Source: CAD feature listing. Evaluate the final solid. Frame: model axes, mm. Give positions to 0.01 mm unless a question says otherwise; leave off trailing zeros. Loops run counter-clockwise (first coordinate to the right, second up) from the corner with the lowest first, then second, coordinate; pieces in that order, holes last. Notation, with made-up numbers: (63.5, 32) - (109.5, 32) arc R28 cw to (109.5, 54) - close; hole circle Ø6 at (-2, 27). An arc over 180 degrees is marked (long way). Write each question's results on one line, items separated by ' | '. Start each with the question number.
(1) Cut plane C-C on x = 182.5. Return the cut outline in (y, z), then the cut area to 3 significant figures.
(2) Cut plane A-A on y = -4. Return the cut outline in (x, z), then the cut area to 3 significant figures.
(3) Material intervals for line 1 along Z through (x, y) = (131, 2.75); line 2 along X through (y, z) = (0.25, -221); line 3 along X through (y, z) = (6.75, -209.5), sorted ascending. Write a range as [from, to].
(4) Cut plane B-B on z = -172. Return the cut outline in (x, y), then the cut area to 3 significant figures.
(5) Contact query for flat-ended pins moving along their axis: pin 1 (5 mm diameter, centred on y = 7, z = -216.5, fed in from +X); pin 2 (3 mm diameter, centred on x = 78, y = 2, fed in from -Z); pin 3 (5 mm diameter, centred on y = 6, z = -40, fed in from -X); pin 4 (8 mm diameter, centred on y = 3.5, z = -171.5, fed in from -X). Output: stop coordinate, or through.
from build123d import *

# Parameters (mm, degrees)
SKETCH1_W           = 220
SKETCH1_H           = 300
BOSS_EXTRUDE1_DEPTH = 10
FILLET1_R           = 30
SKETCH9_W           = 15
SKETCH9_H           = 10
CUT_EXTRUDE1_DEPTH  = 10
SKETCH8_W           = 15
SKETCH8_H           = 10
CUT_EXTRUDE2_DEPTH  = 10
BOSS_EXTRUDE3_DEPTH = 10


with BuildPart() as part:
    # Sketch1 → Boss-Extrude1 (new body)
    with BuildSketch(Plane(origin=(0, 0, 0), x_dir=(1, 0, 0), z_dir=(0, 1, 0))):
        with Locations((110, 150)):
            Rectangle(SKETCH1_W, SKETCH1_H)
    extrude(amount=BOSS_EXTRUDE1_DEPTH)

    # Fillet1
    fillet1_edges = [part.edges().sort_by_distance(p)[0] for p in [
        (0, 5, -300),
        (220, 5, -300),
        (220, 5, 0),
        (0, 5, 0),
    ]]
    fillet(fillet1_edges, radius=FILLET1_R)

    # Sketch9 → Cut-Extrude1 (cut)
    with BuildSketch(Plane(origin=(220, 0, 0), x_dir=(0, 0, -1), z_dir=(1, 0, 0))):
        with Locations((262.5, 5)):
            Rectangle(SKETCH9_W, SKETCH9_H)
        with Locations((232.5, 5)):
            Rectangle(SKETCH9_W, SKETCH9_H)
        with Locations((202.5, 5)):
            Rectangle(SKETCH9_W, SKETCH9_H)
        with Locations((172.5, 5)):
            Rectangle(SKETCH9_W, SKETCH9_H)
        with Locations((142.5, 5)):
            Rectangle(SKETCH9_W, SKETCH9_H)
        with Locations((112.5, 5)):
            Rectangle(SKETCH9_W, SKETCH9_H)
        with Locations((82.5, 5)):
            Rectangle(SKETCH9_W, SKETCH9_H)
        with Locations((52.5, 5)):
            Rectangle(SKETCH9_W, SKETCH9_H)
    extrude(amount=-CUT_EXTRUDE1_DEPTH, mode=Mode.SUBTRACT)

    # Sketch8 → Cut-Extrude2 (cut)
    with BuildSketch(Plane.ZY):
        with Locations((-262.5, 5)):
            Rectangle(SKETCH8_W, SKETCH8_H)
        with Locations((-232.5, 5)):
            Rectangle(SKETCH8_W, SKETCH8_H)
        with Locations((-202.5, 5)):
            Rectangle(SKETCH8_W, SKETCH8_H)
        with Locations((-172.5, 5)):
            Rectangle(SKETCH8_W, SKETCH8_H)
        with Locations((-142.5, 5)):
            Rectangle(SKETCH8_W, SKETCH8_H)
        with Locations((-112.5, 5)):
            Rectangle(SKETCH8_W, SKETCH8_H)
        with Locations((-82.5, 5)):
            Rectangle(SKETCH8_W, SKETCH8_H)
        with Locations((-52.5, 5)):
            Rectangle(SKETCH8_W, SKETCH8_H)
    extrude(amount=-CUT_EXTRUDE2_DEPTH, mode=Mode.SUBTRACT)

    # Sketch11 → Boss-Extrude3 (add)
    with BuildSketch(Plane.XZ):
        with BuildLine():
            Line((229.686269666, -265), (230, -265))
            Line((230, -265), (230, -30))
            ThreePointArc((230, -30), (218.284271247, -1.715728753), (190, 10))
            Line((190, 10), (30, 10))
            ThreePointArc((30, 10), (1.715728753, -1.715728753), (-10, -30))
            Line((-10, -30), (-10, -265))
            Line((-10, -265), (-9.686269666, -265))
            ThreePointArc((-9.686269666, -265), (0, -296.457513111), (30, -310))
            Line((30, -310), (190, -310))
            ThreePointArc((190, -310), (220, -296.457513111), (229.686269666, -265))
        make_face()
    extrude(amount=BOSS_EXTRUDE3_DEPTH)


solid = part.part
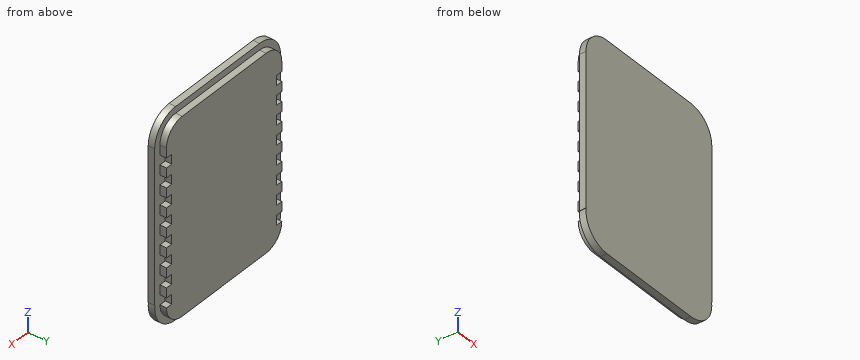
Ans:
1) outline: (-10, -310) - (0, -310) - (0, -300) - (10, -300) - (10, 0) - (0, 0) - (0, 10) - (-10, 10) - close | area: 6,200 mm^2
2) outline: (-10, -265) - (-9.69, -265) arc R40 ccw to (30, -310) - (190, -310) arc R40 ccw to (229.69, -265) - (230, -265) - (230, -30) arc R40 ccw to (190, 10) - (30, 10) arc R40 ccw to (-10, -30) - close | area: 75,400 mm^2
3) line 1: [-300, 0] | line 2: [0, 220] | line 3: [10, 210]
4) outline: (-10, -10) - (230, -10) - (230, 0) - (210, 0) - (210, 10) - (10, 10) - (10, 0) - (-10, 0) - close | area: 4,400 mm^2
5) pin 1: x = 220 | pin 2: z = -300 | pin 3: x = 0 | pin 4: x = -10
